Verification items for this drawing (mm, ordinates from the low corner). A direction names the side the tool comes from. Coordinates: 2 decimals unless noted, no trailing zeros. Loops run counter-clockwise (first coordinate to the right, second up) from the corner with the lowest first, then second, coordinate; pieces in that order, holes last. Notation, with made-up numbers: (-27.5, 52) - (4.5, 52) arc R29 cw to (4.5, 76) - close; hole circle Ø11 at (-8.75, 71.25). An arc over 180 degrees is marked (long way). One line per item, written item: value. Start each with the question number.
(1) Draft check along X on the marked faces 1, 2 and 3. Enter one of: +X half, -X half, draft (parallel to the pull), parting line (faces both ways), or undercut.
(2) Set-up check for the marked faces 4, 5 and 6: record each of +Z, -Z, +X, -X, +Y, -Y from which the full face is reachable in a straight line by a thin tool's end or side.
(3) Section check D-D (z = 5.5). Record the boundary of the cut face in (x, y), plus the area to 3 significant figures.
(4) Thickness scan on probe 1 along X at (y, z) = (5.5, 3.5); probe 2 along X at (y, z) = (4, 15.25); probe 3 along Z at (x, y) = (11, 6.75). Record the ranges inside material, lowest first. Write a range as [from, to].
(5) Section check C-C (y = 5). Record the boundary of the cut face in (x, z), plus the area to 3 significant figures.
(6) Section check B-B (z = 17.25). Record the boundary of the cut face in (x, y), plus the area to 3 significant figures.
(7) Section check A-A (x = 14). Record the boundary of the cut face in (y, z), plus the area to 3 significant figures.
(8) Gauge pin test, flat ends, axial feed: P1, Ø2, axis at y = 7, z = 8.5, coming from the +X side; P2, Ø2, axis at x = 15, y = 5, coming from the +Z side; P3, Ø3, axis at x = 25.5, y = 5.5, coming from the +Z side. Record the tip position at first contact, or that the pin passes through.
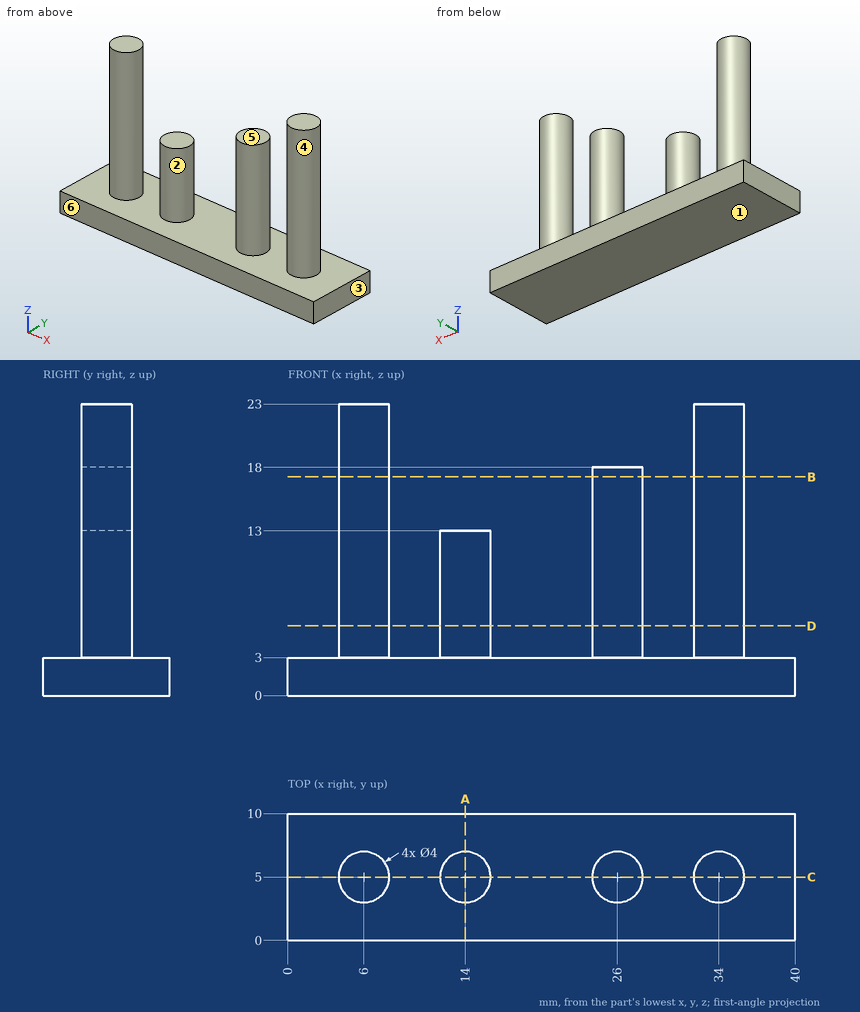
Responses:
1. face 1: draft
1. face 2: undercut
1. face 3: +X half
2. face 4: +Z
2. face 5: +Z, +Y, -Y
2. face 6: +Z, -Z, +X, -X, -Y
3. outline: circle Ø4 at (6, 5); circle Ø4 at (14, 5); circle Ø4 at (26, 5); circle Ø4 at (34, 5)
3. area: 50.3 mm²
4. probe 1: x = [4.06, 7.94], [12.06, 15.94], [24.06, 27.94], [32.06, 35.94]
4. probe 2: x = [4.27, 7.73], [24.27, 27.73], [32.27, 35.73]
4. probe 3: z = [0, 3]
5. outline: (0, 0) - (40, 0) - (40, 3) - (36, 3) - (36, 23) - (32, 23) - (32, 3) - (28, 3) - (28, 18) - (24, 18) - (24, 3) - (16, 3) - (16, 13) - (12, 13) - (12, 3) - (8, 3) - (8, 23) - (4, 23) - (4, 3) - (0, 3) - close
5. area: 380 mm²
6. outline: circle Ø4 at (6, 5); circle Ø4 at (26, 5); circle Ø4 at (34, 5)
6. area: 37.7 mm²
7. outline: (0, 0) - (10, 0) - (10, 3) - (7, 3) - (7, 13) - (3, 13) - (3, 3) - (0, 3) - close
7. area: 70.0 mm²
8. P1: stops at x = 35.73
8. P2: stops at z = 13
8. P3: stops at z = 18
